Can you work these out from the model? Positions are in its coordinate system, mm. A direction names the side the tool comes from. Coordinates: 2 decimals unless noted, no trailing zeros. Order: outer loops, then holes, each group sorted by start corner. A loop starts at its lowest first (then second) coordinate and runs counter-clockwise, first axis right, second up. Notation, with made-up numbers: (28, 41) -> (45, 41) arc R28 cw to (45, 79) -> close; hole circle Ø3 at (56, 12). An arc over 180 degrees is marked (long way). Answer in a Markdown table with one row per item.
```python
from build123d import *

# Parameters (mm, degrees)
SKETCH1_W           = 50.8
SKETCH1_H           = 571.5
BOSS_EXTRUDE1_DEPTH = 12.7
SHELL1_T            = -1.5875
SKETCH5_W           = 31.75
SKETCH5_H           = 26.9875
CUT_EXTRUDE4_DEPTH  = 288.157643987
FILLET2_R           = 3.175
SKETCH3_R           = 2.4892
CUT_EXTRUDE5_DEPTH  = 288.157643987
MIRROR2_START       = 11.1125
MIRROR2_DEPTH       = 1.5875
MIRROR2_START_2     = -25.4
MIRROR2_2_OUTLINE_R = 2.4892
MIRROR2_2_DEPTH     = 50.8


# Read off the part's stored shape, not the designer's step: Mirror2
with BuildPart() as part:
    # Sketch1 → Boss-Extrude1 (new, symmetric)
    with BuildSketch(Plane.XY):
        Rectangle(SKETCH1_W, SKETCH1_H)
    extrude(amount=BOSS_EXTRUDE1_DEPTH, both=True)

    # Shell1
    shell1_openings = [part.faces().sort_by_distance(p)[0] for p in [
        (0, -285.75, 0),
        (0, 285.75, 0),
    ]]
    offset(amount=SHELL1_T, openings=shell1_openings, kind=Kind.INTERSECTION)

    # Sketch5 → Cut-Extrude4 (cut, through all)
    with BuildSketch(Plane.XY):
        with Locations((0, 292.1)):
            Rectangle(SKETCH5_W, SKETCH5_H)
    extrude(amount=CUT_EXTRUDE4_DEPTH, mode=Mode.SUBTRACT)

    # Fillet2
    fillet2_edges = [part.edges().sort_by_distance(p)[0] for p in [
        (15.875, 278.60625, 11.90625),
        (15.875, 285.75, 11.90625),
        (-15.875, 285.75, 11.90625),
        (-15.875, 278.60625, 11.90625),
    ]]
    fillet(fillet2_edges, radius=FILLET2_R)

    # Sketch3 → Cut-Extrude5 (cut, symmetric)
    with BuildSketch(Plane(origin=(0, 0, 0), x_dir=(0, 0, -1), z_dir=(1, 0, 0))):
        with Locations((0, 276.225)):
            Circle(SKETCH3_R)
        with Locations((0, 263.525)):
            Circle(SKETCH3_R)
        with Locations((0, 250.825)):
            Circle(SKETCH3_R)
        with Locations((0, 238.125)):
            Circle(SKETCH3_R)
    extrude(amount=CUT_EXTRUDE5_DEPTH, both=True, mode=Mode.SUBTRACT)

    # Mirror2 outline → Mirror2 (cut)
    with BuildSketch(Plane.XY.offset(MIRROR2_START)):
        with BuildLine():
            Line((-15.875, -285.75), (15.875, -285.75))
            Line((15.875, -285.75), (15.875, -281.78125))
            ThreePointArc((15.875, -281.78125), (14.94506403, -279.53618597), (12.7, -278.60625))
            Line((12.7, -278.60625), (-12.7, -278.60625))
            ThreePointArc((-12.7, -278.60625), (-14.94506403, -279.53618597), (-15.875, -281.78125))
            Line((-15.875, -281.78125), (-15.875, -285.75))
        make_face()
    extrude(amount=MIRROR2_DEPTH, mode=Mode.SUBTRACT)

    # Mirror2 2 outline → Mirror2 2 (cut)
    with BuildSketch(Plane.YZ.offset(MIRROR2_START_2)):
        with Locations((-238.125, 0)):
            Circle(MIRROR2_2_OUTLINE_R)
        with Locations((-250.825, 0)):
            Circle(MIRROR2_2_OUTLINE_R)
        with Locations((-263.525, 0)):
            Circle(MIRROR2_2_OUTLINE_R)
        with Locations((-276.225, 0)):
            Circle(MIRROR2_2_OUTLINE_R)
    extrude(amount=MIRROR2_2_DEPTH, mode=Mode.SUBTRACT)


solid = part.part
```
(1) Suppose I cut it at A-A (x = 4.5). Please give me the cut outline in (y, z).
Response values:
| item | result |
|---|---|
| outline | (-285.75, -12.7) -> (285.75, -12.7) -> (285.75, -11.11) -> (-285.75, -11.11) -> close; (-278.61, 11.11) -> (278.61, 11.11) -> (278.61, 12.7) -> (-278.61, 12.7) -> close |
(2) Suppose I cut it at B-B (y = -75). Please give me the cut outline in (x, z), and give its area (3 significant figures).
Response values:
| item | result |
|---|---|
| outline | (-25.4, -12.7) -> (25.4, -12.7) -> (25.4, 12.7) -> (-25.4, 12.7) -> close; hole (-23.81, -11.11) -> (23.81, -11.11) -> (23.81, 11.11) -> (-23.81, 11.11) -> close |
| area | 232 mm2 |
(3) On a 3-axis mill with a long thin cutter (end or side, diameter ignored), from which of +Z, -Z, +X, -X, +Y, -Y can I reach the whole of each face in a straight line? I mean faces 5 (the flat face through (-2, -285.75, -12)), 6 (the flat face through (0, 4, 11.112)). Say none if no direction works.
Response values:
| item | result |
|---|---|
| face 5 | +Z, -Z, +X, -X, -Y |
| face 6 | +Y, -Y |
(4) We'd pull the mould along Z, two halves only. Please class faces 1 (the flat face through (0, 4, -12.7)), 2 (the flat face through (23.812, -4, 0)), 3 (the flat face through (-25.4, -4, 0)), 4 (the flat face through (0, 4, 12.7)): +Z half, -Z half, draft (parallel to the pull), parting line (faces both ways), or undercut.
Response values:
| item | result |
|---|---|
| face 1 | -Z half |
| face 2 | undercut |
| face 3 | draft |
| face 4 | +Z half |
(5) Will these pins go through, and if not, where does the flat tip stop? pin 1 Ø3 at (y, z) = (-276.225, 0) entering from -X; pin 2 Ø1.7 at (x, z) = (3, 12) entering from +Y; pin 3 Ø0.8 at (x, z) = (-1.5, 12) entering from -Y.
Response values:
| item | result |
|---|---|
| pin 1 | through |
| pin 2 | y = 278.61 |
| pin 3 | y = -278.61 |
(6) I need wall thicknesses on line 1 (Z direction, x = -5, y = -196); line 2 (X direction, y = -195.5, z = 5.75). Which ranges of each line are inside material? Lowest first, please. Write a range as [from, to].
Response values:
| item | result |
|---|---|
| line 1 | [-12.7, -11.11], [11.11, 12.7] |
| line 2 | [-25.4, -23.81], [23.81, 25.4] |
